Geometry check sheet. Reference: the model listing, model coordinates, mm. A direction names the side the tool comes from. Round coordinates to 2 decimals unless told otherwise and drop trailing zeros. Loops run counter-clockwise (first coordinate to the right, second up) from the corner with the lowest first, then second, coordinate; pieces in that order, holes last. Notation, with made-up numbers: M 19.5,-38.75 L 41.5,-38.75 A21 cw 41.5,-11.75 Z; hole C 31.25,86.5 d8. An arc over 180 degrees is marked long. Use one line per item in the form item = value. Start each with the question number.
1. Material ranges on line 1 (Y direction, x = 14, z = 3.75); line 2 (Y direction, x = 19, z = 10); line 3 (Z direction, x = 22, y = -9), recorded low to high.
2. Cross-section at B-B (y = -8.5). Record the boundary of the cut face in (x, z).
3. Cross-section at A-A (y = 0). Record the boundary of the cut face in (x, z).
4. Set-up check for faces 4 (the cylindrical face through (15.947, 0.133, 1.521)), 5 (the flat face through (16, -2, 9.355)): record each of +Z, -Z, +X, -X, +Y, -Y from which the full face is reachable in a straight line by a thin tool's end or side.
5. Cross-section at C-C (z = 7). Record the boundary of the cut face in (x, y), then the cut area to 3 significant figures.
6. Draft check along Z on faces 1 (the cylindrical face through (15.947, 0.133, 10.876)), 2 (the flat face through (18, -10, 6)), 3 (the flat face through (0, 0, 12.355)). Enter one of: pulls with the +Z half, pulls with the -Z half, needs draft (parallel to the pull), parting line crosses it, or undercut.
```python
from build123d import *

# Parameters (mm, degrees)
SKETCH_1_W          = 50
SKETCH_1_H          = 50
EXTRUDE_1_DEPTH     = 12.355487047
SKETCH_2_R          = 3.024908428
CUT_EXTRUDE_1_DEPTH = 15
SKETCH_3_W          = 6.355487047
SKETCH_3_H          = 20
CUT_EXTRUDE_2_DEPTH = 15


with BuildPart() as part:
    # 草图1 → 凸台-拉伸1 (new body)
    with BuildSketch(Plane.XY):
        Rectangle(SKETCH_1_W, SKETCH_1_H)
    extrude(amount=EXTRUDE_1_DEPTH)

    # 草图2 → 切除-拉伸1 (cut)
    with BuildSketch(Plane.XY.offset(12.355487047)):
        with Locations((18.969094387, 0)):
            Circle(SKETCH_2_R)
    extrude(amount=-CUT_EXTRUDE_1_DEPTH, mode=Mode.SUBTRACT)

    # 草图3 → 切除-拉伸2 (cut)
    with BuildSketch(Plane(origin=(25, 0, 0), x_dir=(0, 0, -1), z_dir=(1, 0, 0))):
        with Locations((-6.177743524, 0)):
            Rectangle(SKETCH_3_W, SKETCH_3_H)
    extrude(amount=-CUT_EXTRUDE_2_DEPTH, mode=Mode.SUBTRACT)


solid = part.part
```
Reported:
q1.line_1 = -25 to -10, 10 to 25
q1.line_2 = -25 to -3.02, 3.02 to 25
q1.line_3 = 0 to 3, 9.36 to 12.36
q2.outline = M -25,0 L 25,0 L 25,3 L 10,3 L 10,9.36 L 25,9.36 L 25,12.36 L -25,12.36 Z
q3.outline = M -25,0 L 15.94,0 L 15.94,3 L 10,3 L 10,9.36 L 15.94,9.36 L 15.94,12.36 L -25,12.36 Z; M 21.99,0 L 25,0 L 25,3 L 21.99,3 Z; M 21.99,9.36 L 25,9.36 L 25,12.36 L 21.99,12.36 Z
q4.face_4 = +Z, -Z
q4.face_5 = +X
q5.outline = M -25,-25 L 25,-25 L 25,-10 L 10,-10 L 10,10 L 25,10 L 25,25 L -25,25 Z
q5.area = 2,200 mm²
q6.face_1 = needs draft
q6.face_2 = undercut
q6.face_3 = pulls with the +Z half
